The listing builds one solid part. Answer for the finished solid, in the listing's coordinates (mm). Face numbers are marked on the shaded views. A direction names the side the tool comes from. Give positions to 0.01 mm unless a question says otherwise; leave off trailing zeros. Order: outer loops, then holes, each group sorted by start corner. A loop starts at its lowest first (then second) coordinate and runs counter-clockwise, first axis right, second up. Notation, with made-up numbers: (-4, -38.75) - (2, -38.75) arc R23 ccw to (2, -10.75) - close; hole circle Ø3 at (-37.75, -17). An arc over 180 degrees is marked (long way). Answer as a JSON object with one key per item and string values. Group by question number.
Q1. Given pin 1 (19 mm diameter, centred on x = 38, y = 24.5, fed in from +Z); pin 2 (4 mm diameter, centred on y = 26.5, z = 7.5, fed in from +X); pin 3 (10 mm diameter, centred on y = 12, z = 48.5, fed in from -X), each flat-ended and moving along its own axis, determine where each tip first touches the part or whether it passes through.
Q2. A cutting plane is placed at B-B, the plane x = 7.5. Give the vertices of the cut face in (y, z).
Q3. Consider line 1 (X direction, y = 24, z = 3); line 2 (Z direction, x = 18, y = -27.5); line 3 (X direction, y = -31, z = 8.5). Determine where each line is inside the solid, lowest interval first.
Q4. A cutting plane is placed at C-C, the plane z = 18.5. Give the vertices of the cut face in (x, y).
Q5. A cutting plane is placed at A-A, the plane y = 14.5. Give the vertices of the cut face in (x, z).
Q6. For the marked faces 4, 5 and 6, determine the directions among +Z, -Z, +X, -X, +Y, -Y from which every point of the face is accessible in a straight line to the end or side of a thin tool.
Q7. A cutting plane is placed at D-D, the plane y = -27. Give the vertices of the cut face in (x, z), and give its area (3 significant figures).
Q8. The mould has two halves that part along Z. Classify the marked faces 1, 2 and 3: released by +Z, released by -Z, zero draft, split by the parting line, or undercut.
from build123d import *

# Parameters (mm, degrees)
BOSS_EXTRUDE1_DEPTH = 6
SKETCH3_W           = 30
SKETCH3_H           = 12
BOSS_EXTRUDE2_DEPTH = 9
BOSS_EXTRUDE3_DEPTH = 6
RIB1_START          = -3
RIB1_DEPTH          = 6
RIB2_START          = -3
RIB2_DEPTH          = 6
SKETCH9_R           = 6
CUT_EXTRUDE1_DEPTH  = 6
FILLET1_R           = 12


# Read off the part's stored shape, not the designer's step: Rib1, Rib2
with BuildPart() as part:
    # Sketch1 → Boss-Extrude1 (new body)
    with BuildSketch(Plane.XY):
        Polygon((-50, 36.5), (50, 36.5), (50, -8.5), (3, -36.5), (-3, -36.5), (-50, -8.5), align=None)
    extrude(amount=BOSS_EXTRUDE1_DEPTH)



with BuildPart() as body_2:
    # Sketch3 → Boss-Extrude2 (new body)
    with BuildSketch(Plane.XY.offset(51)):
        with Locations((0, 12.5)):
            Rectangle(SKETCH3_W, SKETCH3_H)
    extrude(amount=-BOSS_EXTRUDE2_DEPTH)


with BuildPart() as part_1:
    add(part.part)

    add(body_2.part)  # Boss-Extrude3 merges body 2
    # Sketch5 → Boss-Extrude3 (add)
    with BuildSketch(Plane(origin=(0, 6.5, 0), x_dir=(-1, 0, 0), z_dir=(0, -1, 0))):
        Polygon((15, -42), (40, -6), (-40, -6), (-15, -42), align=None)
    extrude(amount=-BOSS_EXTRUDE3_DEPTH)

    # Rib1 outline → Rib1 (add)
    with BuildSketch(Plane.ZY.offset(RIB1_START)):
        Polygon((6, -36.5), (51, -5.5), (51, 6.5), (6, 6.5), align=None)
    extrude(amount=RIB1_DEPTH)

    # Rib2 outline → Rib2 (add)
    with BuildSketch(Plane.ZY.offset(RIB2_START)):
        with BuildLine():
            Line((42, 12.5), (42, 18.5))
            Line((42, 18.5), (33.49545417, 18.5))
            ThreePointArc((33.49545417, 18.5), (17.063777445, 23.400199204), (6, 36.5))
            Line((6, 36.5), (6, 12.5))
            Line((6, 12.5), (42, 12.5))
        make_face()
    extrude(amount=RIB2_DEPTH)

    # Sketch9 → Cut-Extrude1 (cut)
    with BuildSketch(Plane.XY):
        with Locations((-38, 24.5)):
            Circle(SKETCH9_R)
        with Locations((38, 24.5)):
            Circle(SKETCH9_R)
    extrude(amount=CUT_EXTRUDE1_DEPTH, mode=Mode.SUBTRACT)

    # Fillet1
    fillet1_edges = [part_1.edges().sort_by_distance(p)[0] for p in [
        (-50, 36.5, 3),
        (50, 36.5, 3),
    ]]
    fillet(fillet1_edges, radius=FILLET1_R)


solid = part_1.part
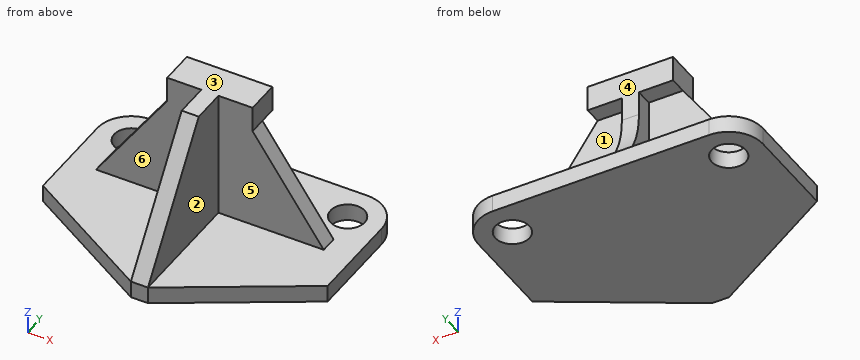
Reply:
{
 "1": {"pin 1": "stops at z = 6", "pin 2": "stops at x = 49.98", "pin 3": "stops at x = -15"},
 "2": {"outline": "(-33.82, 0) - (36.5, 0) - (36.5, 6) - (12.5, 6) - (12.5, 42) - (18.5, 42) - (18.5, 51) - (6.5, 51) - (6.5, 6) - (-33.82, 6) - close"},
 "3": {"line 1": "x = -50 to -43.98, -32.02 to 32.02, 43.98 to 50", "line 2": "z = 0 to 6", "line 3": "x = -3 to 3"},
 "4": {"outline": "(-31.32, 6.5) - (-3, 6.5) - (-3, -27.89) - (3, -27.89) - (3, 6.5) - (31.32, 6.5) - (31.32, 12.5) - (3, 12.5) - (3, 22.52) - (-3, 22.52) - (-3, 12.5) - (-31.32, 12.5) - close"},
 "5": {"outline": "(-50, 0) - (50, 0) - (50, 6) - (3, 6) - (3, 42) - (15, 42) - (15, 51) - (-15, 51) - (-15, 42) - (-3, 42) - (-3, 6) - (-50, 6) - close"},
 "6": {"face 4": "+Z, +X, -X, +Y", "face 5": "+Z, +X, -Y", "face 6": "+Z, -X, -Y"},
 "7": {"outline": "(-18.95, 0) - (18.95, 0) - (18.95, 6) - (3, 6) - (3, 19.79) - (-3, 19.79) - (-3, 6) - (-18.95, 6) - close", "area": "310 mm^2"},
 "8": {"face 1": "undercut", "face 2": "zero draft", "face 3": "released by +Z"}
}
